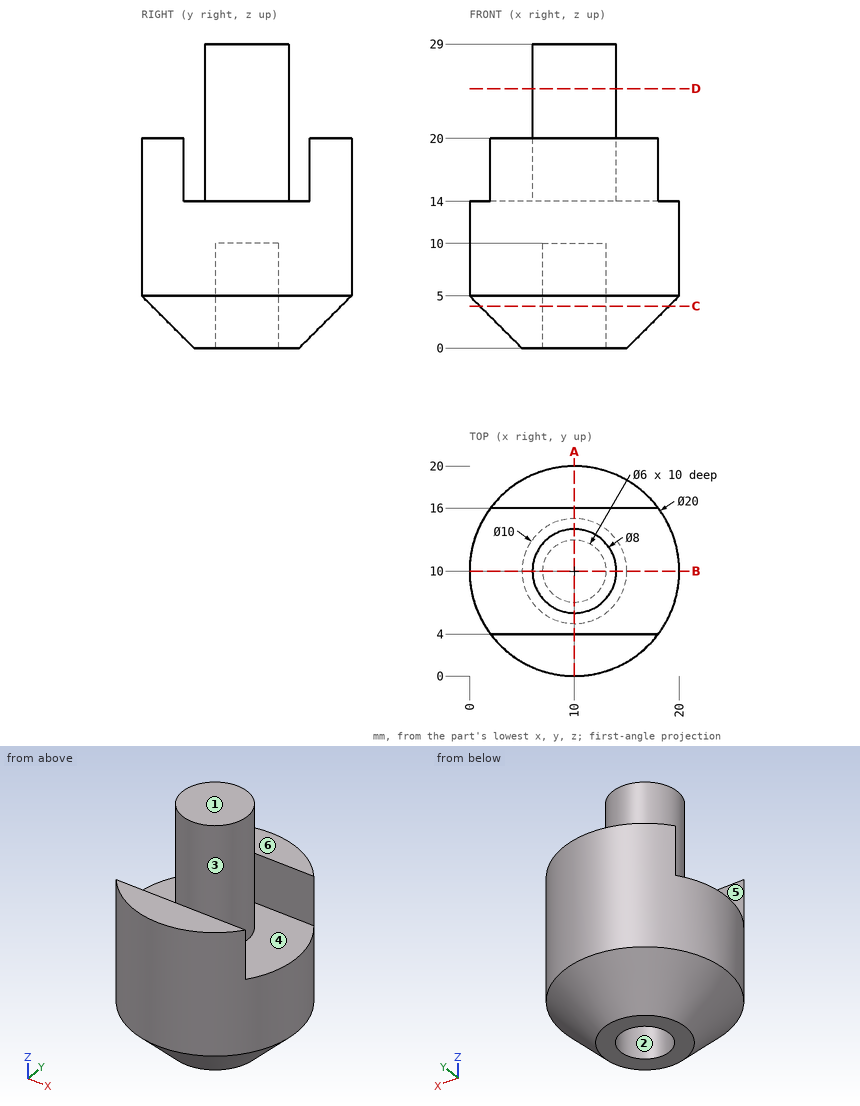
Geometry: see drawing. Coordinates: mm, zero at the bounding-box minimum. A direction names the side the tool comes from. Round coordinates to 2 decimals unless told otherwise and drop trailing zeros. Loops run counter-clockwise (first coordinate to the right, second up) from the corner with the lowest first, then second, coordinate; pieces in that order, holes last. Notation, with made-up numbers: M 49,-0.5 L 72,-0.5 A21 cw 72,3.5 Z; hole C -7,32.5 d3. An arc over 180 degrees is marked long. Use a Markdown table: item, result. Add a question column.
1. Contact query for flat-ended pins moving along their axis: P1, Ø1.8, axis at x = 13, z = 15.5, coming from the +Y side; P2, Ø2, axis at x = 8.5, y = 18.5, coming from the +Z side; P3, Ø4, axis at y = 15.5, z = 3, coming from the +X side. Output: stop coordinate, or through.
2. Section query C-C on z = 4. Return the cut outline in (x, y).
3. Mould query, pull axis X, two halves, no side actions, for the marked faces 1, 2 and 3. Classes: pulls with the +X half, pulls with the -X half, needs draft (parallel to the pull), parting line crosses it, or undercut.
4. Section query B-B on y = 10. Return the cut outline in (x, z).
5. Reachability of the marked faces 4, 5 and 6 from +Z, -Z, +X, -X, +Y, -Y: full face, straight path, thin tool, end or side. Return the list, or none.
6. Line query: line 1 (Y direction, x = 10, z = 7.5); line 2 (Y direction, x = 16, z = 18.75); line 3 (X direction, y = 12.25, z = 8). Output: solid intervals per line, ascending.
7. Section query A-A on x = 10. Return the cut outline in (y, z).
8. Section query D-D on z = 24.75. Return the cut outline in (x, y).
Reported:
| question | item | result |
|---|---|---|
| 1 | P1 | stops at y = 19.78 |
| 1 | P2 | stops at z = 20 |
| 1 | P3 | stops at x = 18.64 |
| 2 | outline | C 10,10 d18; hole C 10,10 d6 |
| 3 | face 1 | needs draft |
| 3 | face 2 | undercut |
| 3 | face 3 | parting line crosses it |
| 4 | outline | M 0,5 L 5,0 L 7,0 L 7,10 L 13,10 L 13,0 L 15,0 L 20,5 L 20,14 L 14,14 L 14,29 L 6,29 L 6,14 L 0,14 Z |
| 5 | face 4 | +Z |
| 5 | face 5 | +Z, +X, -X |
| 5 | face 6 | +Z, +X, -X, +Y |
| 6 | line 1 | y = 0 to 7, 13 to 20 |
| 6 | line 2 | y = 2 to 4, 16 to 18 |
| 6 | line 3 | x = 0.26 to 8.02, 11.98 to 19.74 |
| 7 | outline | M 0,5 L 5,0 L 7,0 L 7,10 L 13,10 L 13,0 L 15,0 L 20,5 L 20,20 L 16,20 L 16,14 L 14,14 L 14,29 L 6,29 L 6,14 L 4,14 L 4,20 L 0,20 Z |
| 8 | outline | C 10,10 d8 |
